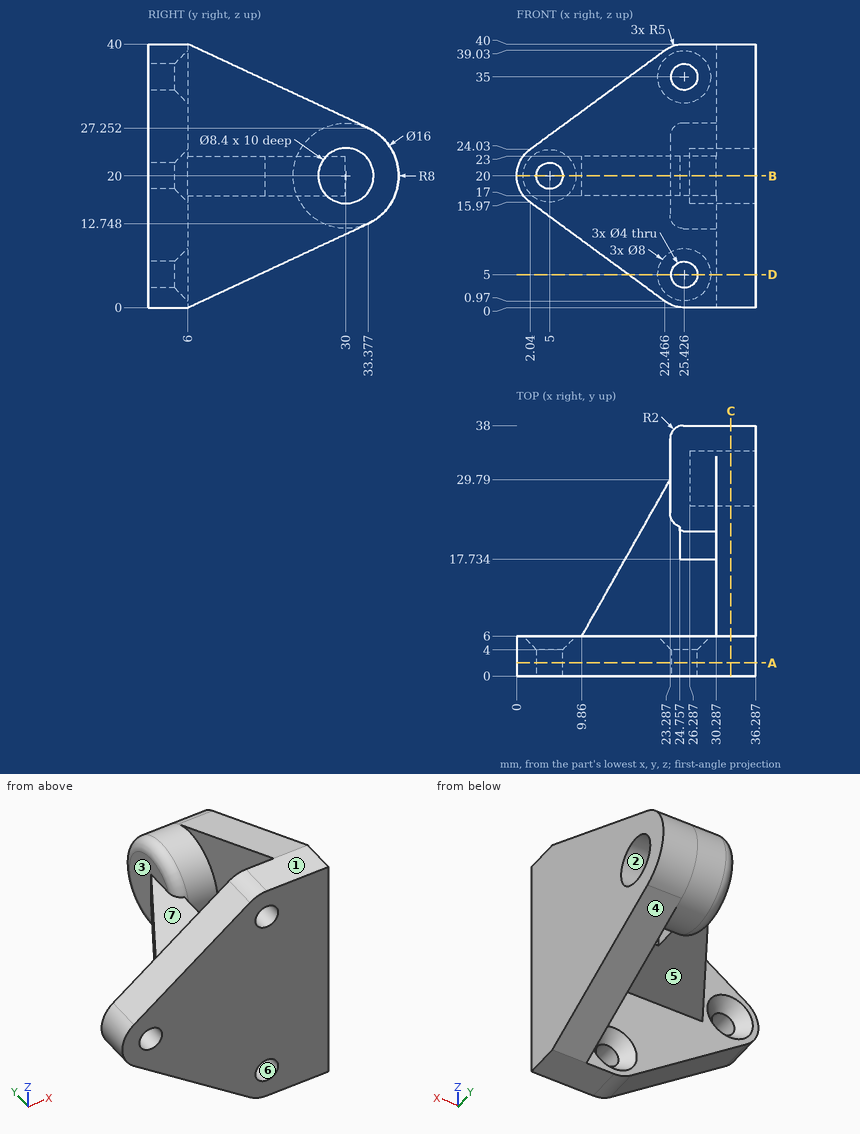
Design review of the part shown in the three views and the two pictorial views. Dimensions are in mm from the part's minimum x, y and z. A direction names the side the tool comes from. Coordinates: 2 decimals unless noted, no trailing zeros. Write each loop counter-clockwise with the first axis right and the second up, starting at its lowest first coordinate (ties: lowest second). Pieces come first, ordered by that corner, then holes.
1) We need section C-C on x = 32.5. State the section outline as (y, z) points, then the cut area to 3 significant figures.
2) The part is to be moulded in two halves that separate along Z. For the marked faces 1, 2, 3 and 4, say which applies: pulls with the +Z half, pulls with the -Z half, needs draft (parallel to the pull), parting line crosses it, or undercut.
3) To check wall thickness, follow probe 1 along Y at (x, z) = (27, 16.5) (1 decimal); probe 2 along Y at (x, z) = (31.5, 20); probe 3 along Y at (x, z) = (22, 38). State the ranges of each line that lie inside material, in increasing order.
4) We need section A-A on y = 2. State the section outline as (x, z) points (1 decimal), then the cut area to 3 significant figures.
5) We need section B-B on z = 20. State the section outline as (x, y) points (1 decimal), then the cut area to 3 significant figures.
6) Clearance check with flat-ended pins moving along their axes: pin 1 Ø5 at (x, z) = (5, 20) entering from +Y; pin 2 Ø16.5 at (x, y) = (21.5, 17) entering from +Z (1 decimal); pin 3 Ø1 at (x, z) = (13, 11.5) entering from +Y; pin 4 Ø3.5 at (x, z) = (25.43, 5) entering from -Y. State where each tip first meets the part, or that it passes through.
7) Machinability: for the marked faces 5, 6 and 7, which of the approach directions +Z, -Z, +X, -X, +Y, -Y give a long, thin tool a straight path to every point of the face, cutting with its end or side? Answer none if there is none.
8) We need section D-D on z = 5. State the section outline as (x, y) points (1 decimal).
Answer list:
1. outline: (0, 0) - (6, 0) - (33.38, 12.75) arc R8 ccw to (33.38, 27.25) - (6, 40) - (0, 40) - close; hole circle Ø8.4 at (30, 20)
1. area: 979 mm2
2. face 1: pulls with the +Z half
2. face 2: undercut
2. face 3: needs draft
2. face 4: pulls with the -Z half
3. probe 1: y = 0 to 6, 22.8 to 27.7, 32.3 to 37.2
3. probe 2: y = 0 to 25.8, 34.2 to 38
3. probe 3: y = 0 to 6
4. outline: (2, 16) - (22.5, 1) arc R5 ccw to (25.4, 0) - (36.3, 0) - (36.3, 40) - (25.4, 40) arc R5 ccw to (22.5, 39) - (2, 24) arc R5 ccw to start; hole circle Ø4 at (5, 20); hole circle Ø4 at (25.4, 5); hole circle Ø4 at (25.4, 35)
4. area: 996 mm2
5. outline: (0, 0) - (3, 0) - (3, 4) - (1, 6) - (0, 6) - close; (7, 0) - (36.3, 0) - (36.3, 25.8) - (26.3, 25.8) - (26.3, 34.2) - (36.3, 34.2) - (36.3, 38) - (25.3, 38) arc R2 ccw to (23.3, 36) - (23.3, 29.8) - (9.9, 6) - (9, 6) - (7, 4) - close; hole (24.8, 17.7) - (30.3, 17.7) - (30.3, 22) - (25.3, 22) arc R2 cw to (24.8, 22.1) - close
5. area: 657 mm2
6. pin 1: stops at y = 4.5
6. pin 2: stops at z = 25.8
6. pin 3: stops at y = 6
6. pin 4: passes through
7. face 5: -Z, -X
7. face 6: +Y, -Y
7. face 7: +Z, -X
8. outline: (17, 0) - (23.4, 0) - (23.4, 4) - (21.4, 6) - (17, 6) - close; (27.4, 0) - (36.3, 0) - (36.3, 16.7) - (30.3, 16.7) - (30.3, 6) - (29.4, 6) - (27.4, 4) - close
